Here's how the part is built. I have some questions about the finished solid (model axes, mm). A direction names the side the tool comes from. Round coordinates to 2 decimals unless told otherwise and drop trailing zeros. Order: outer loops, then holes, each group sorted by start corner. A loop starts at its lowest first (then second) coordinate and runs counter-clockwise, first axis right, second up. Notation, with made-up numbers: (22, 53) -> (51, 53) arc R24 ccw to (51, 76) -> close; hole circle Ø11 at (3.25, 16). An arc over 180 degrees is marked (long way). Use a Markdown table: item, result. Add a question column.
(1) I want a section at A-A, the plane z = 13. Please give me the cut outline in (x, y).
(2) I want a section at B-B, the plane x = -40. Please give me the cut outline in (y, z).
(3) On a 3-axis mill with a long thin cutter (end or side, diameter ignored), from which of +Z, -Z, +X, -X, +Y, -Y can I reach the whole of each face in a straight line? I mean faces 1 (the face through (-1, 8, -31)), 2 (the face through (-4, 7, 34)), 3 (the face through (0, 7, -32)). Say none if no direction works.
(4) I'm going to push flat-ended pins straight in: P1, Ø18.5, axis at x = 19.5, z = 8.5, coming from the +Y side; P2, Ø3, axis at x = -1, y = 6, coming from the -Z side; P3, Ø1.2, axis at x = -1, z = 33, coming from the -Y side; P4, Ø1.3, axis at x = 0, z = -34, coming from the +Y side. Where does each tip first touch, or does it pass through?
(5) If I drill on probe 1 along Z at (x, y) = (63, 11.25); probe 2 along X at (y, z) = (4, -28); probe 3 along Y at (x, z) = (-21, -10), over which ranges is the centre line in solid material (lowest first)?
(6) Thinking about a two-plate mould opening in X: for faces 4 (the face through (84.1, 8.07, 35.14)), 5 (the face through (0, 13, -32)), 6 (the face through (-4.16, 0.86, 32.89)), which applies, pulls with the +X half, pulls with the -X half, needs draft (parallel to the pull), parting line crosses it, or undercut?
from build123d import *

# Parameters (mm, degrees)
SKETCH_1_W          = 170
SKETCH_1_H          = 72
EXTRUDE_1_DEPTH     = 3
SKETCH_2_W          = 170
SKETCH_2_H          = 72
SKETCH_2_W_2        = 165
SKETCH_2_H_2        = 62
EXTRUDE_2_DEPTH     = 10
CUT_EXTRUDE_1_DEPTH = 10.5
SKETCH_5_R          = 1.05
CUT_EXTRUDE_2_DEPTH = 10.5
SKETCH_6_R          = 1.05
CUT_EXTRUDE_3_DEPTH = 10.5
FILLET_1_R          = 3


with BuildPart() as part:
    # 草图1 → 凸台-拉伸1 (new body)
    with BuildSketch(Plane(origin=(0, 0, 0), x_dir=(1, 0, 0), z_dir=(0, 1, 0))):
        Rectangle(SKETCH_1_W, SKETCH_1_H)
    extrude(amount=EXTRUDE_1_DEPTH)

    # 草图2 → 凸台-拉伸2 (add)
    with BuildSketch(Plane(origin=(0, 3, 0), x_dir=(1, 0, 0), z_dir=(0, 1, 0))):
        Rectangle(SKETCH_2_W, SKETCH_2_H)
        Rectangle(SKETCH_2_W_2, SKETCH_2_H_2, mode=Mode.SUBTRACT)
    extrude(amount=EXTRUDE_2_DEPTH)

    # 草图3 → 切除-拉伸1 (cut)
    with BuildSketch(Plane.XZ):
        Polygon((-6, 36), (-2, 32), (2, 32), (6, 36), align=None)
        Polygon((6, -36), (-6, -36), (-2, -32), (2, -32), align=None)
    extrude(amount=-CUT_EXTRUDE_1_DEPTH, mode=Mode.SUBTRACT)

    # 草图5 → 切除-拉伸2 (cut)
    with BuildSketch(Plane.XZ.offset(-10.5)):
        with Locations(Location((0, 34, 0), (0, 0, 270))):
            Circle(SKETCH_5_R)
    extrude(amount=-CUT_EXTRUDE_2_DEPTH, mode=Mode.SUBTRACT)

    # 草图6 → 切除-拉伸3 (cut)
    with BuildSketch(Plane.XZ.offset(-10.5)):
        with Locations(Location((0, -34, 0), (0, 0, 270))):
            Circle(SKETCH_6_R)
    extrude(amount=-CUT_EXTRUDE_3_DEPTH, mode=Mode.SUBTRACT)

    # 圆角1
    fillet_1_edges = [part.edges().sort_by_distance(p)[0] for p in [
        (45.5, 0, 36),
        (-45.5, 0, -36),
        (-4, 0, 34),
        (0, 0, 32),
        (4, 0, 34),
        (-45.5, 0, 36),
        (4, 0, -34),
        (0, 0, -32),
        (-85, 0, 0),
        (-4, 0, -34),
        (45.5, 0, -36),
        (85, 0, 0),
        (85, 6.5, 36),
        (-85, 6.5, 36),
        (-85, 6.5, -36),
        (85, 6.5, -36),
    ]]
    fillet(fillet_1_edges, radius=FILLET_1_R)


solid = part.part
Taken from the geometry:
| question | item | result |
|---|---|---|
| 1 | outline | (-85, 3) arc R3 ccw to (-82, 0) -> (82, 0) arc R3 ccw to (85, 3) -> (85, 13) -> (82.5, 13) -> (82.5, 3) -> (-82.5, 3) -> (-82.5, 13) -> (-85, 13) -> close |
| 2 | outline | (0, -33) arc R3 ccw to (3, -36) -> (13, -36) -> (13, -31) -> (3, -31) -> (3, 31) -> (13, 31) -> (13, 36) -> (3, 36) arc R3 ccw to (0, 33) -> close |
| 3 | face 1 | +Y |
| 3 | face 2 | +Z, -Y |
| 3 | face 3 | -Z, -Y |
| 4 | P1 | stops at y = 3 |
| 4 | P2 | stops at z = -32.5 |
| 4 | P3 | stops at y = 10.5 |
| 4 | P4 | passes through |
| 5 | probe 1 | z = -36 to -31, 31 to 36 |
| 5 | probe 2 | x = -85 to -82.5, 82.5 to 85 |
| 5 | probe 3 | y = 0 to 3 |
| 6 | face 4 | pulls with the +X half |
| 6 | face 5 | needs draft |
| 6 | face 6 | undercut |
